Autodesk Inventor part; units mm, degrees
ref_plane "YZ Plane" through (0, 0, 0) normal (1, 0, 0) x (0, 1, 0)
ref_plane "XZ Plane" through (0, 0, 0) normal (0, 1, 0) x (-1, 0, 0)
ref_plane "XY Plane" through (0, 0, 0) normal (0, 0, 1) x (1, 0, 0)
sketch "Sketch1" plane through (0, 0, 0) normal (0, 0, 1) x (1, 0, 0)
  line L0 (-247.5, 247.5) -> (247.5, 247.5)
  line L1 (247.5, 247.5) -> (247.5, -247.5)
  line L2 (247.5, -247.5) -> (-247.5, -247.5)
  line L3 (-247.5, -247.5) -> (-247.5, 247.5)
  line L4 (-247.5, -247.5) -> (247.5, 247.5) construction
  point P0 (0, 0)
  point P1 (0, 0)
  dimension "d0" = 495
  dimension "d1" = 495
extrude "Extrusion1" add sketch "Sketch1" against normal blind 10
sketch "Sketch2" plane through (0, 0, -10) normal (0, 0, -1) x (-1, 0, 0)
  line L0 (197.5, -197.5) -> (-197.5, -197.5)
  line L1 (-197.5, -197.5) -> (-197.5, 197.5)
  line L2 (-197.5, 197.5) -> (197.5, 197.5)
  line L3 (197.5, 197.5) -> (197.5, -197.5)
  line L4 (197.5, -197.5) -> (-197.5, 197.5) construction
  line L5 (247.5, -247.5) -> (247.5, 247.5)
  line L6 (197.5, -197.5) -> (247.5, -197.5)
  line L7 (247.5, -197.5) -> (247.5, -187.5)
  line L8 (247.5, -187.5) -> (197.5, -187.5)
  line L9 (197.5, -187.5) -> (197.5, -197.5)
  line L10 (197.5, 197.5) -> (247.5, 197.5)
  line L11 (247.5, 197.5) -> (247.5, 187.5)
  line L12 (247.5, 187.5) -> (197.5, 187.5)
  line L13 (197.5, 187.5) -> (197.5, 197.5)
  line L14 (-247.5, 247.5) -> (-247.5, -247.5)
  line L15 (-197.5, -197.5) -> (-247.5, -197.5)
  line L16 (-247.5, -197.5) -> (-247.5, -187.5)
  line L17 (-247.5, -187.5) -> (-197.5, -187.5)
  line L18 (-197.5, -187.5) -> (-197.5, -197.5)
  line L19 (-197.5, 197.5) -> (-247.5, 197.5)
  line L20 (-247.5, 197.5) -> (-247.5, 187.5)
  line L21 (-247.5, 187.5) -> (-197.5, 187.5)
  line L22 (-197.5, 187.5) -> (-197.5, 197.5)
  point P0 (0, 0)
  point P1 (0, 0)
  dimension "d4" = 395
  dimension "d5" = 395
  dimension "d19" = 10
  dimension "d20" = 10
  dimension "d21" = 10
  dimension "d22" = 10
extrude "Extrusion2" add sketch "Sketch2" along normal blind 320 contours L0 L1 L2 L3 | L3 L8 L5 L6 | L15 L14 L17 L1 | L3 L10 L5 L12 | L21 L14 L19 L1
sketch "Sketch3" plane through (0, 0, -330) normal (0, 0, -1) x (-1, 0, 0)
  line L0 (-247.5, -247.5) -> (247.5, -247.5)
  line L1 (247.5, -247.5) -> (247.5, 247.5)
  line L2 (247.5, 247.5) -> (-247.5, 247.5)
  line L3 (-247.5, 247.5) -> (-247.5, -247.5)
  line L4 (-247.5, -247.5) -> (247.5, 247.5) construction
  point P0 (0, 0)
  point P1 (0, 0)
  dimension "d8" = 495
  dimension "d9" = 495
extrude "Extrusion3" add sketch "Sketch3" along normal blind 10
sketch "Sketch4" plane through (0, 0, 0) normal (0, 0, 1) x (1, 0, 0)
  line L0 (-187.5, -187.5) -> (187.5, -187.5)
  line L1 (187.5, -187.5) -> (187.5, 187.5)
  line L2 (187.5, 187.5) -> (-187.5, 187.5)
  line L3 (-187.5, 187.5) -> (-187.5, -187.5)
  line L4 (-187.5, -187.5) -> (187.5, 187.5) construction
  point P0 (0, 0)
  point P1 (0, 0)
  dimension "d12" = 375
  dimension "d13" = 375
extrude "Extrusion4" cut sketch "Sketch4" against normal through all
sketch "Sketch6" plane through (-247.5, -197.5, -10) normal (0, -1, 0) x (1, 0, 0)
  line L0 (235, -42.5) -> (405, -42.5)
  line L1 (405, -42.5) -> (405, -247.5)
  line L2 (405, -247.5) -> (235, -247.5)
  line L3 (235, -247.5) -> (235, -42.5)
  line L4 (235, -42.5) -> (405, -247.5) construction
  line L5 (495, 0) -> (495, -320)
  line L6 (495, -330) -> (0, -330)
  point P0 (247.5, 10)
  point P1 (320, -145)
  dimension "d23" = 205
  dimension "d24" = 170
  dimension "d25" = 175
  dimension "d26" = 185
extrude "Extrusion5" add sketch "Sketch6" along normal blind 220
sketch "Sketch7" plane through (-12.5, -197.5, -257.5) normal (-1, 0, 0) x (0, 0, 1)
  circle A0 centre (160, -165) radius 125
  line L0 (205, 0) -> (205, -220)
  line L1 (205, -220) -> (0, -220)
  point P0 (257.5, 197.5)
  dimension "d5" = 395
  dimension "d30" = 250
  dimension "d33" = 45
  dimension "d34" = 55
extrude "Extrusion6" add sketch "Sketch7" along normal blind 27
sketch "Sketch8" plane through (-39.5, -362.5, -97.5) normal (-1, 0, 0) x (0, 0, 1)
  circle A0 centre (0, 0) radius 97.5
  circle A1 centre (0, 0) radius 125
  point P0 (97.5, 362.5)
  dimension "d37" = 195
extrude "Extrusion7" add sketch "Sketch8" along normal blind 292 contours A0
pattern_circular "Circular Pattern1" count 2 over 360 about axis through (0, 0, -10) along (0, 0, 1) of "Extrusion7", "Extrusion6", "Extrusion5"
sketch "Sketch10" plane through (-197.5, -187.5, -10) normal (-1, 0, 0) x (0, 0, 1)
  line L0 (-77.5, 363.5) -> (-242.5, 363.5)
  line L1 (-242.5, 363.5) -> (-242.5, 276.5)
  line L2 (-242.5, 276.5) -> (-77.5, 276.5)
  line L3 (-77.5, 276.5) -> (-77.5, 363.5)
  line L4 (0, 375) -> (-320, 375)
  point P0 (10, 187.5)
  point P1 (-77.5, 320)
  point P2 (-160, 363.5)
  point P3 (-160, 375)
  dimension "d44" = 165
  dimension "d45" = 87
  dimension "d46" = 55
extrude "Extrusion8" add sketch "Sketch10" along normal blind 125
chamfer "Chamfer1" distance 30 angle 45 2 edges at (-322.5, 132.5, -87.5) (-322.5, 132.5, -252.5)
chamfer "Chamfer2" distance 30 angle 45 2 edges at (331.5, 362.5, -195) (-331.5, -362.5, -195)
equation "\"d1\" = d0"
equation "\"d5\" = d4"
equation "\"d20\" = d19"
equation "\"d21\" = d19"
equation "\"d22\" = d19"
equation "\"d8\" = d0"
equation "\"d9\" = d8"
properties part number "Измельчитель комков"
CAD build for the part. Positions are in the model's coordinates, mm. A direction names the side the tool comes from. Round coordinates to 2 decimals unless told otherwise and drop trailing zeros. Loops run counter-clockwise (first coordinate to the right, second up) from the corner with the lowest first, then second, coordinate; pieces in that order, holes last. Notation, with made-up numbers: (89.25, 38.25) - (130.25, 38.25) arc R32 cw to (130.25, 64.25) - close; hole circle Ø9 at (9, 75.5). An arc over 180 degrees is marked (long way). Return JSON: item names as keys, results as strings. Group by question number.
Q1. Two-plate mould, pull along Y, no slides. Class faces 6 (the face through (3, 223, -330)), 7 (the face through (197.5, -3, -168)): +Y half, -Y half, draft (parallel to the pull), parting line (faces both ways), or undercut.
Q2. Tool access for faces 1 (the face through (-3, -222, -10)), 2 (the face through (25.81, 446.98, -189.63)), 3 (the face through (3, 187.5, -168)), 4 (the face through (71, -306, -52.5)), 5 (the face through (-244, 132, -87.5)): list every direction of +Z, -Z, +X, -X, +Y, -Y with a clear straight run to the whole face (end or side of a thin tool).
Q3. Band-saw the part on D-D on z = -303.5. Give the cut face in (x, y), plus the area to 3 significant figures.
Q4. Flat gauge pins, fed straight in: pin 1 Ø12 at (y, z) = (324.5, -197) entering from -X; pin 2 Ø25 at (x, z) = (233, -182.5) entering from +Y; pin 3 Ø6 at (x, y) = (233, -20.5) entering from +Z. Where does each tip first touch, or does it go through?
Q5. Band-saw the part on B-B on x = 230. Give the cut face in (y, z), plus the area to 3 significant figures.
Q6. Band-saw the part on A-A on x = 62. Give the cut face in (y, z).
Q7. Band-saw the part on C-C on y = -362.5. Give the cut face in (x, z), plus the area to 3 significant figures.
Q8. Drill centre lines: line 1 along Y through (x, z) = (125, -201); line 2 along Y through (x, z) = (-245, -248); line 3 along Y through (x, z) = (29, -169). Where is each one in solid material? Low to high. Write a range as [from, to].
Solutions:
{
 "1": {"face 6": "draft", "face 7": "undercut"},
 "2": {"face 1": "+X, -X", "face 2": "+X", "face 3": "+Z, -Z", "face 4": "+X, -Y", "face 5": "-X"},
 "3": {"outline": "(-247.5, -197.5) - (247.5, -197.5) - (247.5, -187.5) - (197.5, -187.5) - (197.5, 187.5) - (247.5, 187.5) - (247.5, 197.5) - (-247.5, 197.5) - (-247.5, 187.5) - (-197.5, 187.5) - (-197.5, -187.5) - (-247.5, -187.5) - close; hole (-187.5, -187.5) - (187.5, -187.5) - (187.5, 187.5) - (-187.5, 187.5) - close", "area": "17,400 mm^2"},
 "4": {"pin 1": "stops at x = -157.5", "pin 2": "stops at y = 427.69", "pin 3": "stops at z = 0"},
 "5": {"outline": "(-247.5, -340) - (247.5, -340) - (247.5, -330) - (197.5, -330) - (197.5, -10) - (247.5, -10) - (247.5, 0) - (-247.5, 0) - (-247.5, -10) - (-197.5, -10) - (-197.5, -330) - (-247.5, -330) - close; circle Ø195 at (362.5, -97.5); hole (-187.5, -330) - (187.5, -330) - (187.5, -10) - (-187.5, -10) - close", "area": "46,200 mm^2"},
 "6": {"outline": "(-417.5, -257.5) - (-197.5, -257.5) - (-197.5, -330) - (-247.5, -330) - (-247.5, -340) - (-187.5, -340) - (-187.5, 0) - (-247.5, 0) - (-247.5, -10) - (-197.5, -10) - (-197.5, -52.5) - (-417.5, -52.5) - close; (187.5, -340) - (247.5, -340) - (247.5, -330) - (197.5, -330) - (197.5, -10) - (247.5, -10) - (247.5, 0) - (187.5, 0) - close; circle Ø195 at (362.5, -97.5)"},
 "7": {"outline": "(-331.5, -165) - (-301.5, -195) - (-39.5, -195) - (-39.5, -222.5) - (-12.5, -222.5) - (-12.5, -257.5) - (157.5, -257.5) - (157.5, -52.5) - (-12.5, -52.5) - (-12.5, 27.5) - (-39.5, 27.5) - (-39.5, 0) - (-301.5, 0) - (-331.5, -30) - close", "area": "97,600 mm^2"},
 "8": {"line 1": "y = [-417.5, -187.5], [187.5, 197.5]", "line 2": "y = [-197.5, -187.5], [89, 176], [187.5, 197.5]", "line 3": "y = [-417.5, -187.5], [187.5, 197.5], [259.97, 465.03]"}
}
